from build123d import *

# Parameters (mm, degrees)
SKETCH2_R           = 5.5
BOSS_EXTRUDE1_DEPTH = 8
SKETCH3_R           = 1.1
CUT_EXTRUDE1_DEPTH  = 40.752358421
CUT_EXTRUDE2_START  = -8
SKETCH5_R           = 1.75
CUT_EXTRUDE2_DEPTH  = 88
SKETCH6_R           = 1.1
CUT_EXTRUDE3_DEPTH  = 40.752358441
FILLET2_R           = 8
FILLET1_R           = 1


with BuildPart() as part:
    # Sketch2 → Boss-Extrude1 (new body)
    with BuildSketch(Plane.XY):
        with BuildLine():
            Line((0, -38), (3, -38))
            Line((3, -38), (3, -7.95298686))
            ThreePointArc((3, -7.95298686), (0, 8.5), (-3, -7.95298686))
            Line((-3, -7.95298686), (-3, -38))
            Line((-3, -38), (0, -38))
        make_face()
        Circle(SKETCH2_R, mode=Mode.SUBTRACT)
    extrude(amount=BOSS_EXTRUDE1_DEPTH)

    # Sketch3 → Cut-Extrude1 (cut, through all)
    with BuildSketch(Plane(origin=(0, 0, 0), x_dir=(1, 0, 0), z_dir=(0, 1, 0))):
        with Locations(Location((0, -4, 0), (0, 0, 270))):
            Circle(SKETCH3_R)
    extrude(amount=-CUT_EXTRUDE1_DEPTH, mode=Mode.SUBTRACT)

    # Sketch5 → Cut-Extrude2 (cut)
    with BuildSketch(Plane(origin=(0, 0, 0), x_dir=(1, 0, 0), z_dir=(0, 1, 0)).offset(CUT_EXTRUDE2_START)):
        with Locations(Location((0, -4, 0), (0, 0, 270))):
            Circle(SKETCH5_R)
    extrude(amount=-CUT_EXTRUDE2_DEPTH, mode=Mode.SUBTRACT)

    # Sketch6 → Cut-Extrude3 (cut, through all)
    with BuildSketch(Plane(origin=(0, 0, 0), x_dir=(0, 0, -1), z_dir=(1, 0, 0))):
        with Locations((-4, 0)):
            Circle(SKETCH6_R)
    extrude(amount=-CUT_EXTRUDE3_DEPTH, mode=Mode.SUBTRACT)

    # Fillet2
    fillet2_edges = [part.edges().sort_by_distance(p)[0] for p in [
        (3, -7.95298686, 4),
        (-3, -7.95298686, 4),
    ]]
    fillet(fillet2_edges, radius=FILLET2_R)

    # Fillet1
    fillet1_edges = [part.edges().sort_by_distance(p)[0] for p in [
        (0, -38, 8),
        (3, -25.149186938, 8),
        (0, 8.5, 0),
        (0, 8.5, 8),
        (-3, -25.149186938, 0),
        (-3, -25.149186938, 8),
        (3.697032567, -9.032387553, 0),
        (3.697032567, -9.032387553, 8),
        (-3.697032567, -9.032387553, 0),
        (-3.697032567, -9.032387553, 8),
        (3, -25.149186938, 0),
        (0, -38, 0),
        (3, -38, 4),
        (-3, -38, 4),
    ]]
    fillet(fillet1_edges, radius=FILLET1_R)


solid = part.part
For this review, take the finished solid that the model builds, in its own axes (mm). A direction names the side the tool comes from. Give positions to 0.01 mm unless a question says otherwise; leave off trailing zeros. Order: outer loops, then holes, each group sorted by start corner. A loop starts at its lowest first (then second) coordinate and runs counter-clockwise, first axis right, second up. Notation, with made-up numbers: (-24.75, 67.5) - (9.25, 67.5) arc R24 ccw to (9.25, 90.5) - close; hole circle Ø5 at (23.5, 68.5). An arc over 180 degrees is marked (long way). Answer as a JSON object with one key per item and string values. Group by question number.
Item 1: Machinability: for faces 1 (the flat face through (-3, -24, 4)), 2 (the cylindrical face through (-0.421, -6.676, 5.016)), 3 (the cylindrical face through (-2.699, -24.822, 0.285)), which of the approach directions +Z, -Z, +X, -X, +Y, -Y give a long, thin tool a straight path to every point of the face, cutting with its end or side? Answer none if there is none.
Item 2: Take a section at B-B on y = -15.5. Give the boundary of the cut face in (x, z).
Item 3: Clearance check with flat-ended pins moving along their axes: pin 1 Ø1.8 at (y, z) = (-29.5, 5.5) entering from -X; pin 2 Ø3 at (y, z) = (-32, 4) entering from +X; pin 3 Ø2 at (x, y) = (4, 1.5) entering from -Z; pin 4 Ø1.8 at (x, z) = (0.5, 4.5) entering from -Y. State where each tip first meets the part, or that it passes through.
Item 4: Draft analysis for pull direction X (two halves, no side actions). For faces 4 (the flat face through (-1, -8, 3)), 5 (the cylindrical face through (-2.699, -37.715, 4.042)), 6 (the cylindrical face through (2.715, -24.476, 7.699)), 7 (the flat face through (1.3, -38, 2.6)), state which applies: pulls with the +X half, pulls with the -X half, needs draft (parallel to the pull), parting line crosses it, or undercut.
Item 5: Take a section at C-C on z = 3.75. Give the boundary of the cut face in (x, y).
Item 6: Take a section at D-D on y = 0. Give the number of separate pieces and of enclosed holes in the cut face, and give its area (3 significant figures).
Item 7: Wall thickness on line 1 along Y through (x, z) = (0, 5.25); line 2 along Z through (x, y) = (0, -6); line 3 along X through (y, z) = (-29.5, 4): over which ranges is each line inside the solid? List them lowest first.
Item 8: Take a section at A-A on x = 0. Give the boundary of the cut face in (y, z).
Reported:
{
 "1": {"face 1": "+Z, -Z, -X, -Y", "face 2": "-Y", "face 3": "-Z, -X, -Y"},
 "2": {"outline": "(-3, 1) arc R1 ccw to (-2, 0) - (2, 0) arc R1 ccw to (3, 1) - (3, 7) arc R1 ccw to (2, 8) - (-2, 8) arc R1 ccw to (-3, 7) - close; hole circle Ø3.5 at (0, 4)"},
 "3": {"pin 1": "x = -3", "pin 2": "x = 3", "pin 3": "through", "pin 4": "y = -8"},
 "4": {"face 4": "undercut", "face 5": "pulls with the -X half", "face 6": "pulls with the +X half", "face 7": "needs draft"},
 "5": {"outline": "(-8.43, -1.07) arc R8.5 ccw to (-5.67, -6.34) arc R8 cw to (-3, -12.3) - (-3, -37) arc R1 ccw to (-2, -38) - (-1.73, -38) - (-1.73, -8) - (-1.07, -8) - (-1.07, -5.39) arc R5.5 cw to (-5.39, -1.07) - close; (-8.43, 1.07) - (-5.39, 1.07) arc R5.5 cw (long way) to (1.07, -5.39) - (1.07, -8) - (1.73, -8) - (1.73, -38) - (2, -38) arc R1 ccw to (3, -37) - (3, -12.3) arc R8 cw to (5.67, -6.34) arc R8.5 ccw (long way) to start"},
 "6": {"separate pieces": "3", "enclosed holes": "0", "area": "40.5 mm^2"},
 "7": {"line 1": "-8 to -5.5, 5.5 to 8.5", "line 2": "0 to 2.9, 5.1 to 8", "line 3": "-3 to -1.75, 1.75 to 3"},
 "8": {"outline": "(-38, 1) arc R1 ccw to (-37, 0) - (-5.5, 0) - (-5.5, 2.9) - (-8, 2.9) - (-8, 2.25) - (-38, 2.25) - close; (-38, 5.75) - (-8, 5.75) - (-8, 5.1) - (-5.5, 5.1) - (-5.5, 8) - (-37, 8) arc R1 ccw to (-38, 7) - close; (5.5, 0) - (7.5, 0) arc R1 ccw to (8.5, 1) - (8.5, 7) arc R1 ccw to (7.5, 8) - (5.5, 8) - close"}
}
